Here's how the part is built. I have some questions about the finished solid (model axes, mm). A direction names the side the tool comes from. Give positions to 0.01 mm unless a question says otherwise; leave off trailing zeros. Loops run counter-clockwise (first coordinate to the right, second up) from the corner with the lowest first, then second, coordinate; pieces in that order, holes last.
Q1. Will these pins go through, and if not, where does the flat tip stop? P1, Ø10, axis at x = 15.5, y = -12.5, coming from the +Z side; P2, Ø4, axis at y = -41, z = 14, coming from the -X side; P3, Ø6, axis at y = -13, z = 4, coming from the -X side.
Q2. I need wall thicknesses on line 1 (Z direction, x = -9, y = -14); line 2 (Z direction, x = -12.5, y = -44); line 3 (X direction, y = -6.5, z = 4). Which ranges of each line are inside material? Lowest first, please.
Q3. For faces 4 (the face through (-5.876, -24.653, 10.01)), 5 (the face through (-7.04, -0.06, 12.55)), 6 (the face through (-5.965, -0.057, 10.342)), 7 (the face through (-16, -25, 0)), which set-ups out of +Z, -Z, +X, -X, +Y, -Y let a thin tool reach every point of the face, with its end or its side?
Q4. If we section it at A-A (x = 15): Please give me the cut outline in (y, z).
Q5. If we section it at B-B (y = -15): Please give me the cut outline in (x, z).
Q6. We'd pull the mould along Z, two halves only. Please class faces 1 (the face through (-7.04, -49.94, 12.55)), 2 (the face through (0, -25, -1)), 3 (the face through (15, -25, 0)): +Z half, -Z half, draft (parallel to the pull), parting line (faces both ways), or undercut.
from build123d import *

# Parameters (mm, degrees)
F1_DEPTH    = 50
F2_R        = 5
F3_R        = 0.6
F4_R        = 0.2
F5_T1_DEPTH = 50.516331174
F5_T3_DEPTH = 50.6913085011


# Not quite as in the source:
# - a fillet or chamfer that OpenCascade refuses, or shapes differently, is made with other operations: its cross-section is extruded or revolved along the edge and cut away or added


with BuildPart() as f1:
    # F0 (on Front) → F1 (new body)
    with BuildSketch(Plane.XZ):
        Polygon((5, 0), (-5, 0), (-6.743114855, 19.9238939618), (-7.743114855, 19.9238939618), (-6, 0), (-20, 0), (-21, -1), (21, -1), (20, 0), (6, 0), (4.256885145, 19.9238939618), (3.256885145, 19.9238939618), align=None)
    extrude(amount=F1_DEPTH)

    # F2
    f2_edges = [f1.edges().sort_by_distance(p)[0] for p in [
        (-6, -25, 0),
        (6, -25, 0),
    ]]
    fillet(f2_edges, radius=F2_R)

    # F3
    f3_edges = [f1.edges().sort_by_distance(p)[0] for p in [
        (-5, -25, 0),
        (5, -25, 0),
    ]]
    fillet(f3_edges, radius=F3_R)

    # F4
    f4_edges = [f1.edges().sort_by_distance(p)[0] for p in [
        (-21, -25, -1),
        (21, -25, -1),
        (0, 0, -1),
        (0, -50, -1),
        (-5.895516, -50, 10.2358),
        (-4.855555, -50, 0.157634),
        (-7.243115, -50, 19.923894),
        (-0.052493, -50, 0),
        (-7.109342, -50, 12.679836),
        (4.787581, -50, 0.194646),
        (-7.770156, -50, 1.622049),
        (4.099908, -50, 10.288094),
        (-15.728271, -50, 0),
        (3.756885, -50, 19.923894),
        (-20.5, -50, -0.5),
        (4.928784, -50, 12.244058),
        (7.203705, -50, 1.313613),
        (20.5, -50, -0.5),
        (15.290828, -50, 0),
        (-5.895516, 0, 10.2358),
        (-4.855555, 0, 0.157634),
        (-7.243115, 0, 19.923894),
        (-0.052493, 0, 0),
        (-7.109342, 0, 12.679836),
        (4.787581, 0, 0.194646),
        (-7.770156, 0, 1.622049),
        (4.099908, 0, 10.288094),
        (-15.728271, 0, 0),
        (3.756885, 0, 19.923894),
        (-20.5, 0, -0.5),
        (4.928784, 0, 12.244058),
        (7.203705, 0, 1.313613),
        (20.5, 0, -0.5),
        (15.290828, 0, 0),
    ]]
    fillet(f4_edges, radius=F4_R)

    # F5: fillet of radius 0.2 on 8 edges, made by hand

    # F5_s2 → F5_t1 (cut)
    with BuildSketch(Plane.XZ.offset(-0.258165587)):
        with BuildLine():
            ThreePointArc((-6.9263810898, 19.9238939618), (-6.7912630482, 19.8713494292), (-6.7271421501, 19.7413251104))
            Line((-6.7271421501, 19.7413251104), (-6.743114855, 19.9238939618))
            Line((-6.743114855, 19.9238939618), (-6.9263810898, 19.9238939618))
        make_face()
        with BuildLine():
            ThreePointArc((4.2728578499, 19.7413251104), (4.2087369518, 19.8713494292), (4.0736189102, 19.9238939618))
            Line((4.0736189102, 19.9238939618), (4.256885145, 19.9238939618))
            Line((4.256885145, 19.9238939618), (4.2728578499, 19.7413251104))
        make_face()
    extrude(amount=F5_T1_DEPTH, mode=Mode.SUBTRACT)

    # F5_s4 → F5_t3 (cut)
    with BuildSketch(Plane.XZ.offset(-0.3456542505)):
        with BuildLine():
            ThreePointArc((-7.7240920944, 19.7064628133), (-7.6723086221, 19.8590120034), (-7.5248531547, 19.9238939618))
            Line((-7.5248531547, 19.9238939618), (-7.743114855, 19.9238939618))
            Line((-7.743114855, 19.9238939618), (-7.7240920944, 19.7064628133))
        make_face()
        with BuildLine():
            ThreePointArc((3.4751468453, 19.9238939618), (3.3276913779, 19.8590120034), (3.2759079056, 19.7064628133))
            Line((3.2759079056, 19.7064628133), (3.256885145, 19.9238939618))
            Line((3.256885145, 19.9238939618), (3.4751468453, 19.9238939618))
        make_face()
    extrude(amount=F5_T3_DEPTH, mode=Mode.SUBTRACT)


solid = f1.part
Check sheet entries:
1. P1: stops at z = 0
1. P2: stops at x = -7.4
1. P3: stops at x = -8.46
2. line 1: z = -1 to 0.65
2. line 2: z = -1 to 0
2. line 3: x = -6.56 to -5.35, 4.65 to 5.68
3. face 4: +Z, +Y, -Y
3. face 5: -X, +Y
3. face 6: +Z, +Y
3. face 7: +Z, -X, +Y, -Y
4. outline: (-50, -0.8) arc R0.2 ccw to (-49.8, -1) - (-0.2, -1) arc R0.2 ccw to (0, -0.8) - (0, -0.2) arc R0.2 ccw to (-0.2, 0) - (-49.8, 0) arc R0.2 ccw to (-50, -0.2) - close
5. outline: (-20.66, -0.66) arc R0.2 ccw to (-20.52, -1) - (20.52, -1) arc R0.2 ccw to (20.66, -0.66) - (20, 0) - (10.58, 0) arc R5 cw to (5.6, 4.56) - (4.27, 19.74) arc R0.2 ccw to (4.07, 19.92) - (3.48, 19.92) arc R0.2 ccw to (3.28, 19.71) - (4.94, 0.65) arc R0.6 cw to (4.35, 0) - (-4.45, 0) arc R0.6 cw to (-5.05, 0.55) - (-6.73, 19.74) arc R0.2 ccw to (-6.93, 19.92) - (-7.52, 19.92) arc R0.2 ccw to (-7.72, 19.71) - (-6.48, 5.44) arc R5 cw to (-11.46, 0) - (-20, 0) - close
6. face 1: undercut
6. face 2: -Z half
6. face 3: +Z half
